from build123d import *

# Parameters (mm, degrees)
BOSS_EXTRUDE1_DEPTH = 3.81
SKETCH2_W           = 1.806317066
SKETCH2_H           = 1.967276013
SKETCH2_W_2         = 1.806317067
BOSS_EXTRUDE3_DEPTH = 8.8


with BuildPart() as part:
    # Sketch1 → Boss-Extrude1 (new body)
    with BuildSketch(Plane(origin=(0, 0, 0), x_dir=(1, 0, 0), z_dir=(0, 1, 0))):
        Polygon((36.52712799, -14.326641718), (36.52712799, -62.609481683), (-60.401431987, -62.609481683), (-60.401431987, 42.143358282), (-9.091431987, 42.143358282), (-5.281431987, 42.143358282), (-5.281431987, 38.333358282), (-5.281431987, -10.233061701), (32.71712799, -10.516641718), (36.52712799, -10.516641718), align=None)
    extrude(amount=BOSS_EXTRUDE1_DEPTH)

    # Sketch2 → Boss-Extrude3 (add)
    with BuildSketch(Plane(origin=(0, 3.81, 0), x_dir=(1, 0, 0), z_dir=(0, 1, 0))):
        with Locations((34.771422609, -12.560052875)):
            Rectangle(SKETCH2_W, SKETCH2_H)
        with Locations((-7.268072139, 40.235776176)):
            Rectangle(SKETCH2_W_2, SKETCH2_H)
        with Locations((-58.508052472, 39.991804454)):
            Rectangle(SKETCH2_W_2, SKETCH2_H)
        with Locations((-58.311142754, -60.507662725)):
            Rectangle(SKETCH2_W_2, SKETCH2_H)
        with Locations((34.614322263, -60.589626835)):
            Rectangle(SKETCH2_W, SKETCH2_H)
    extrude(amount=-BOSS_EXTRUDE3_DEPTH)


solid = part.part
Here's how the part is built. I have some questions about the finished solid (model axes, mm). A direction names the side the tool comes from. Give positions to 0.01 mm unless a question says otherwise; leave off trailing zeros. Loops run counter-clockwise (first coordinate to the right, second up) from the corner with the lowest first, then second, coordinate; pieces in that order, holes last. Notation, with made-up numbers: (65.25, 68) -> (105.25, 68) arc R26 cw to (105.25, 93) -> close; hole circle Ø10 at (35.25, 15.25). An arc over 180 degrees is marked (long way). Answer as a JSON object with one key per item and string values. Group by question number.
Item 1: On a 3-axis mill with a long thin cutter (end or side, diameter ignored), from which of +Z, -Z, +X, -X, +Y, -Y can I reach the whole of each face in a straight line? I mean faces 1 (the flat face through (-60.401, 2, 11)), 2 (the flat face through (-5.281, 2, -16)). Say none if no direction works.
Item 2: I need wall thicknesses on L1, parallel to Y at x = -22, z = -34; L2, parallel to Z at x = -8, y = -0.5; L3, parallel to X at y = 1.25, z = -30. Which ranges of each line are inside material? Lowest first, please.
Item 3: Imagine slicing it at A-A on y = -3.25. Write out the boundary of the cut face in (x, z).
Item 4: Imagine slicing it at C-C on x = -39.5. Write out the boundary of the cut face in (y, z).
Item 5: Imagine slicing it at B-B on z = 19. Write out the boundary of the cut face in (x, y), then the cut area to 3 significant figures.
Item 6: Will these pins go through, and if not, where does the flat tip stop? pin 1 (5 mm diameter, centred on x = -30, y = -3, fed in from +Z) (1 decimal); pin 2 (0.5 mm diameter, centred on x = -58.5, y = -1.5, fed in from -Z); pin 3 (0.9 mm diameter, centred on x = -7.5, y = -2.5, fed in from -Z); pin 4 (1.6 mm diameter, centred on y = -3, z = -40, fed in from -X).
Answer list:
{
 "1": {"face 1": "+Z, -Z, -X, +Y, -Y", "face 2": "-Z, +X, +Y, -Y"},
 "2": {"L1": "y = 0 to 3.81", "L2": "z = -41.22 to -39.25", "L3": "x = -60.4 to -5.28"},
 "3": {"outline": "(-59.41, -40.98) -> (-57.6, -40.98) -> (-57.6, -39.01) -> (-59.41, -39.01) -> close; (-59.21, 59.52) -> (-57.41, 59.52) -> (-57.41, 61.49) -> (-59.21, 61.49) -> close; (-8.17, -41.22) -> (-6.36, -41.22) -> (-6.36, -39.25) -> (-8.17, -39.25) -> close; (33.71, 59.61) -> (35.52, 59.61) -> (35.52, 61.57) -> (33.71, 61.57) -> close; (33.87, 11.58) -> (35.67, 11.58) -> (35.67, 13.54) -> (33.87, 13.54) -> close"},
 "4": {"outline": "(0, -42.14) -> (3.81, -42.14) -> (3.81, 62.61) -> (0, 62.61) -> close"},
 "5": {"outline": "(-60.4, 0) -> (36.53, 0) -> (36.53, 3.81) -> (-60.4, 3.81) -> close", "area": "369 mm2"},
 "6": {"pin 1": "passes through", "pin 2": "stops at z = -40.98", "pin 3": "stops at z = -41.22", "pin 4": "stops at x = -59.41"}
}
